For this review, use the dimensioned drawing (mm, ordinates from the lowest corner) and the shaded views. Coordinates: 2 decimals unless noted, no trailing zeros. Order: outer loops, then holes, each group sorted by start corner. A loop starts at its lowest first (then second) coordinate and runs counter-clockwise, first axis right, second up. Notation, with made-up numbers: M 17.5,-30.5 L 65.5,-30.5 A21 ccw 65.5,4.5 Z; hole C 4.5,84.5 d1. An arc over 180 degrees is marked long. One line per item, written item: value.
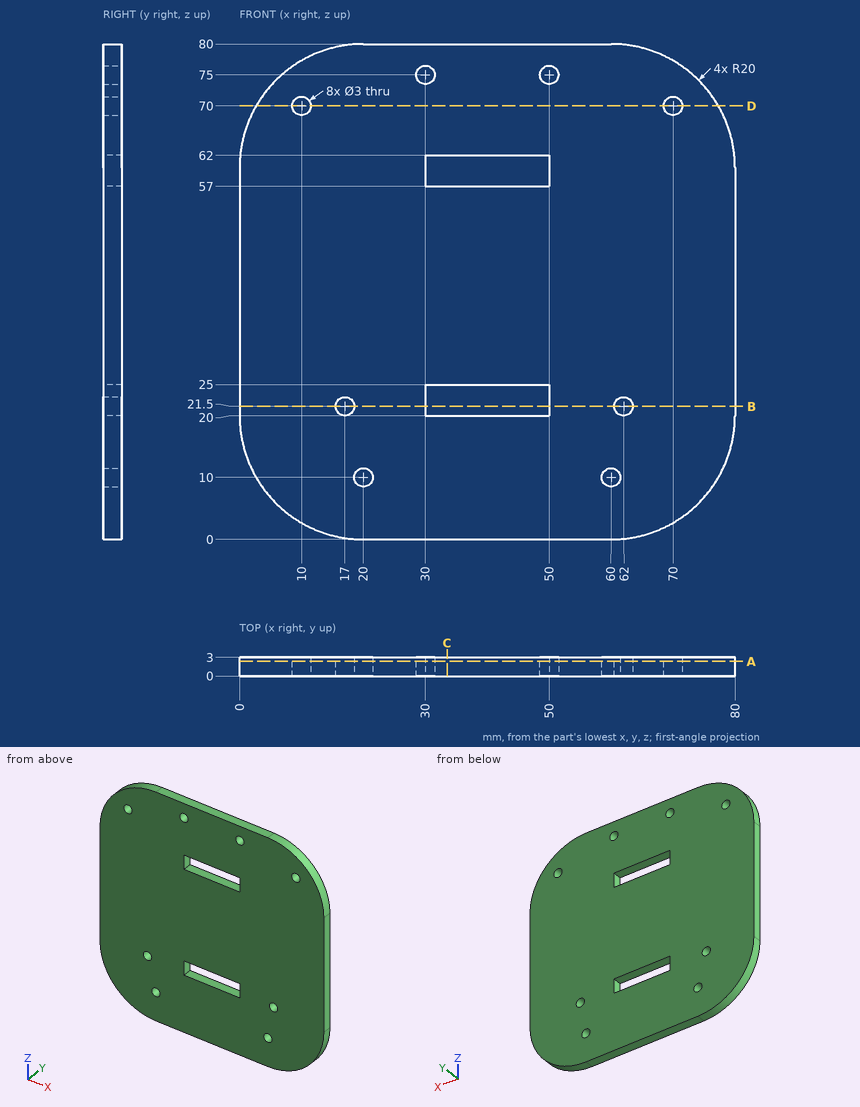
(1) For L1, parallel to Z at x = 39, y = 0.55; L2, parallel to X at y = 2.3, z = 21.5; L3, parallel to X at y = 1.45, z = 75, list the stretches that pass through material, from the lowest coordinate up.
Geometry results:
L1: z = 0 to 20, 25 to 57, 62 to 80
L2: x = 0 to 15.5, 18.5 to 30, 50 to 60.5, 63.5 to 80
L3: x = 6.77 to 28.5, 31.5 to 48.5, 51.5 to 73.23
(2) We need section D-D, the plane z = 70. State the section outline as (x, y) points, plus the area to 3 significant figures.
Geometry results:
outline: M 2.68,0 L 8.5,0 L 8.5,3 L 2.68,3 Z; M 11.5,0 L 68.5,0 L 68.5,3 L 11.5,3 Z; M 71.5,0 L 77.32,0 L 77.32,3 L 71.5,3 Z
area: 206 mm2
(3) Insertion check: pin 1 Ø1.5 at (y, z) = (2.5, 61) entering from +X. The pin has a flat end and moves straight along its axis. Give the tip position at first contact, or say it passes through.
Geometry results:
pin 1: stops at x = 80
(4) We need section C-C, the plane x = 33.5. State the section outline as (y, z) points.
Geometry results:
outline: M 0,0 L 3,0 L 3,20 L 0,20 Z; M 0,25 L 3,25 L 3,57 L 0,57 Z; M 0,62 L 3,62 L 3,80 L 0,80 Z
(5) We need section A-A, the plane y = 2.35. Count the separate pieces of the cut face and the enclosed holes in it, plus the area to 3 significant figures.
Geometry results:
separate pieces: 1
enclosed holes: 10
area: 5,800 mm2
(6) We need section B-B, the plane z = 21.5. State the section outline as (x, y) points, plus the area to 3 significant figures.
Geometry results:
outline: M 0,0 L 15.5,0 L 15.5,3 L 0,3 Z; M 18.5,0 L 30,0 L 30,3 L 18.5,3 Z; M 50,0 L 60.5,0 L 60.5,3 L 50,3 Z; M 63.5,0 L 80,0 L 80,3 L 63.5,3 Z
area: 162 mm2
